Could you check a few things on this model? Use its own coordinates, in mm. A direction names the side the tool comes from. Give positions to 0.01 mm unless a question says otherwise; leave off trailing zeros. Order: outer loops, then holes, each group sorted by start corner. A loop starts at its lowest first (then second) coordinate and runs counter-clockwise, first axis right, second up.
from build123d import *

# Parameters (mm, degrees)
SKETCH_1_W                  = 220
SKETCH_1_H                  = 220
EXTRUDE_1_DEPTH             = 20
EXTRUDE_1_TAPER             = 45
SKETCH_2_W                  = 8
SKETCH_2_H                  = 20
EXTRUDE_2_DEPTH             = 30
EXTRUDE_2_DIRECTION_2_REACH = 158.844
SKETCH_4_W                  = 220
SKETCH_4_H                  = 220
EXTRUDE_3_DEPTH             = 30
CUT_EXTRUDE_1_DEPTH         = 15
SKETCH_7_R                  = 90
CUT_EXTRUDE_2_DEPTH         = 28
SKETCH_9_R                  = 5
CUT_EXTRUDE_3_DEPTH         = 5
CUT_EXTRUDE_4_DEPTH         = 251.99800796
PATTERN_CIRCULAR_2_COUNT    = 4


with BuildPart() as part:
    # 스케치1 → 보스-돌출1 (new body)
    with BuildSketch(Plane.XY):
        Rectangle(SKETCH_1_W, SKETCH_1_H)
    extrude(amount=EXTRUDE_1_DEPTH, taper=EXTRUDE_1_TAPER)

    # 스케치2 → 보스-돌출2 (add)
    with BuildSketch(Plane.XY.offset(20)):
        with Locations((-81, 60)):
            Rectangle(SKETCH_2_W, SKETCH_2_H)
        with Locations((-81, -60)):
            Rectangle(SKETCH_2_W, SKETCH_2_H)
        with Locations((81, 85)):
            Rectangle(SKETCH_2_W, SKETCH_2_H)
        with Locations((81, -85)):
            Rectangle(SKETCH_2_W, SKETCH_2_H)
    extrude(amount=EXTRUDE_2_DEPTH)

    # 보스-돌출2 direction 2: up to this face of the body (flat: up to its plane)
    extrude_2_direction_2_end = Plane(part.part.faces().sort_by_distance((0, 0, 0))[0])
    # 스케치2 → 보스-돌출2 direction 2 (add, up to the picked face)
    with BuildSketch(Plane.XY.offset(20), mode=Mode.PRIVATE) as extrude_2_direction_2_sk1:
        with Locations((-81, 60)):
            Rectangle(SKETCH_2_W, SKETCH_2_H)
    extrude_2_direction_2_tool1 = split(extrude(extrude_2_direction_2_sk1.sketch, amount=-EXTRUDE_2_DIRECTION_2_REACH, mode=Mode.PRIVATE), bisect_by=extrude_2_direction_2_end, keep=Keep.BOTH, mode=Mode.PRIVATE)
    # 스케치2 → 보스-돌출2 direction 2 (add, up to the picked face)
    with BuildSketch(Plane.XY.offset(20), mode=Mode.PRIVATE) as extrude_2_direction_2_sk2:
        with Locations((-81, -60)):
            Rectangle(SKETCH_2_W, SKETCH_2_H)
    extrude_2_direction_2_tool2 = split(extrude(extrude_2_direction_2_sk2.sketch, amount=-EXTRUDE_2_DIRECTION_2_REACH, mode=Mode.PRIVATE), bisect_by=extrude_2_direction_2_end, keep=Keep.BOTH, mode=Mode.PRIVATE)
    # 스케치2 → 보스-돌출2 direction 2 (add, up to the picked face)
    with BuildSketch(Plane.XY.offset(20), mode=Mode.PRIVATE) as extrude_2_direction_2_sk3:
        with Locations((81, 85)):
            Rectangle(SKETCH_2_W, SKETCH_2_H)
    extrude_2_direction_2_tool3 = split(extrude(extrude_2_direction_2_sk3.sketch, amount=-EXTRUDE_2_DIRECTION_2_REACH, mode=Mode.PRIVATE), bisect_by=extrude_2_direction_2_end, keep=Keep.BOTH, mode=Mode.PRIVATE)
    # 스케치2 → 보스-돌출2 direction 2 (add, up to the picked face)
    with BuildSketch(Plane.XY.offset(20), mode=Mode.PRIVATE) as extrude_2_direction_2_sk4:
        with Locations((81, -85)):
            Rectangle(SKETCH_2_W, SKETCH_2_H)
    extrude_2_direction_2_tool4 = split(extrude(extrude_2_direction_2_sk4.sketch, amount=-EXTRUDE_2_DIRECTION_2_REACH, mode=Mode.PRIVATE), bisect_by=extrude_2_direction_2_end, keep=Keep.BOTH, mode=Mode.PRIVATE)
    add(extrude_2_direction_2_tool1.solids().sort_by(Axis((-81, 60, 20), (0, 0, -1)))[0])
    add(extrude_2_direction_2_tool2.solids().sort_by(Axis((-81, -60, 20), (0, 0, -1)))[0])
    add(extrude_2_direction_2_tool3.solids().sort_by(Axis((81, 85, 20), (0, 0, -1)))[0])
    add(extrude_2_direction_2_tool4.solids().sort_by(Axis((81, -85, 20), (0, 0, -1)))[0])

    # 스케치4 → 보스-돌출3 (add)
    with BuildSketch(Plane(origin=(0, 0, 0), x_dir=(-1, 0, 0), z_dir=(0, 0, -1))):
        Rectangle(SKETCH_4_W, SKETCH_4_H)
    extrude(amount=EXTRUDE_3_DEPTH)

    # 스케치6 → 컷-돌출1 (cut)
    with BuildSketch(Plane(origin=(0, 0, -23), x_dir=(-1, 0, 0), z_dir=(0, 0, -1))):
        with BuildLine():
            Line((-110, 25), (-75, 25))
            ThreePointArc((-75, 25), (-60.355339059, 60.355339059), (-25, 75))
            Line((-25, 75), (-25, 110))
            Line((-25, 110), (25, 110))
            Line((25, 110), (25, 75))
            ThreePointArc((25, 75), (60.355339059, 60.355339059), (75, 25))
            Line((75, 25), (110, 25))
            Line((110, 25), (110, -25))
            Line((110, -25), (75, -25))
            ThreePointArc((75, -25), (60.355339059, -60.355339059), (25, -75))
            Line((25, -75), (25, -110))
            Line((25, -110), (-25, -110))
            Line((-25, -110), (-25, -75))
            ThreePointArc((-25, -75), (-60.355339059, -60.355339059), (-75, -25))
            Line((-75, -25), (-110, -25))
            Line((-110, -25), (-110, 25))
        make_face()
    extrude(amount=-CUT_EXTRUDE_1_DEPTH, mode=Mode.SUBTRACT)

    # 스케치7 → 컷-돌출2 (cut)
    with BuildSketch(Plane.XY.offset(20)):
        Circle(SKETCH_7_R)
    extrude(amount=-CUT_EXTRUDE_2_DEPTH, mode=Mode.SUBTRACT)

    # 스케치9 → 컷-돌출3 (cut)
    with BuildSketch(Plane.XY.offset(-23)):
        with Locations((-35, 35)):
            Circle(SKETCH_9_R)
        Circle(SKETCH_9_R)
        with Locations((35, 35)):
            Circle(SKETCH_9_R)
        with Locations(Location((35, -35, 0), (0, 0, 180))):
            Circle(SKETCH_9_R)
        with Locations(Location((-35, -35, 0), (0, 0, 180))):
            Circle(SKETCH_9_R)
    extrude(amount=-CUT_EXTRUDE_3_DEPTH, mode=Mode.SUBTRACT)

    # 스케치10 → 컷-돌출4 (cut, through all)
    with BuildSketch(Plane(origin=(0, 110, 0), x_dir=(1, 0, 0), z_dir=(0, 1, 0))):
        Polygon((-110, 30), (-110, 27.5), (-107.5, 30), align=None)
    cut_extrude_4 = extrude(amount=-CUT_EXTRUDE_4_DEPTH, mode=Mode.SUBTRACT)

    # 원형 패턴2: 컷-돌출4 ×4 about axis
    pattern_circular_2_axis = Axis((0, 0, 0), (0, 0, 1))
    for i in range(1, PATTERN_CIRCULAR_2_COUNT):
        add(cut_extrude_4.rotate(pattern_circular_2_axis, i * 360 / PATTERN_CIRCULAR_2_COUNT), mode=Mode.SUBTRACT)


solid = part.part
Item 1: Imagine slicing it at A-A on x = -94. List the corners of the cut face in (y, z) for me, then the cut area to 3 significant figures.
Findings:
outline: (-110, -27.5) - (-107.5, -30) - (107.5, -30) - (110, -27.5) - (110, 0) - (94, 16) - (-94, 16) - (-110, 0) - close; hole (-25, -23) - (25, -23) - (25, -8) - (-25, -8) - close
area: 9,110 mm2
Item 2: Imagine slicing it at C-C on x = 21.5. List the corners of the cut face in (y, z) for me.
Findings:
outline: (-110, -27.5) - (-107.5, -30) - (107.5, -30) - (110, -27.5) - (110, -23) - (-110, -23) - close; (-110, -8) - (-87.39, -8) - (-87.39, 20) - (-90, 20) - (-110, 0) - close; (87.39, -8) - (110, -8) - (110, 0) - (90, 20) - (87.39, 20) - close
Item 3: We'd pull the mould along Z, two halves only. Please class faces 5 (the flat face through (-25, 93, -16)), 6 (the flat face through (100, 2, 10)), 7 (the cylindrical face through (-60.742, -59.964, -15.605)): +Z half, -Z half, draft (parallel to the pull), parting line (faces both ways), or undercut.
Findings:
face 5: undercut
face 6: +Z half
face 7: draft
Item 4: Imagine slicing it at B-B on z = 42.5. List the corners of the cut face in (x, y) for me, then the cut area to 3 significant figures.
Findings:
outline: (-85, -70) - (-77, -70) - (-77, -50) - (-85, -50) - close; (-85, 50) - (-77, 50) - (-77, 70) - (-85, 70) - close; (77, -95) - (85, -95) - (85, -75) - (77, -75) - close; (77, 75) - (85, 75) - (85, 95) - (77, 95) - close
area: 640 mm2
Item 5: For faces 1 (the cylindrical face through (41.53, -79.845, 6.196)), 2 (the flat face through (81, -75, 35)), 3 (the flat face through (93, 25, -16)), 4 (the flat face through (-85, -60, 35)), which set-ups out of +Z, -Z, +X, -X, +Y, -Y let a thin tool reach every point of the face, with its end or its side?
Findings:
face 1: +Z
face 2: +Z, +X, -X
face 3: +X, -X
face 4: +Z, -X, +Y, -Y
Item 6: For pin 1 (6 mm diameter, centred on y = 22.5, z = 18.5, fed in from -X); pin 2 (3 mm diameter, centred on x = -2, y = -1.5, fed in from +Z); pin 3 (13 mm diameter, centred on x = 35, y = -35, fed in from +Z), each with a flat end and sliding along its axis, tell me the tip position at first contact or that it passes through.
Findings:
pin 1: stops at x = -94.5
pin 2: stops at z = -28
pin 3: stops at z = -23
Item 7: Please list where these lines run through material, in increasing order: line 1 along X through (y, z) = (-35, -25.55); line 2 along Y through (x, z) = (98, -9).
Findings:
line 1: x = -110 to -40, -30 to 30, 40 to 110
line 2: y = -110 to -25, 25 to 110
Item 8: Imagine slicing it at D-D on y = -17. List the corners of the cut face in (x, z) for me.
Findings:
outline: (-110, -27.5) - (-107.5, -30) - (107.5, -30) - (110, -27.5) - (110, -23) - (-110, -23) - close; (-110, -8) - (-88.38, -8) - (-88.38, 20) - (-90, 20) - (-110, 0) - close; (88.38, -8) - (110, -8) - (110, 0) - (90, 20) - (88.38, 20) - close
